Geometry: final body of the model. Coordinates: model frame, mm. A direction names the side the tool comes from. Give positions to 0.01 mm unless a question says otherwise; leave off trailing zeros. Loops run counter-clockwise (first coordinate to the right, second up) from the corner with the lowest first, then second, coordinate; pieces in that order, holes last. Notation, with made-up numbers: (-6, 65.25) -> (0, 65.25) arc R18 ccw to (0, 73.25) -> close; hole circle Ø5 at (6.5, 26.25). An arc over 180 degrees is marked (long way). Answer in a Markdown table with one row per item. Add a question column.
1) First-contact query: P1, Ø18, axis at x = -15.5, y = 5.5, coming from the +Z side; P2, Ø9.5, axis at y = -6, z = 10, coming from the +X side; P3, Ø2, axis at y = -13.5, z = 29, coming from the -X side; P4, Ø1.2, axis at x = -25.5, y = 16, coming from the +Z side. Flat tips, straight axial feed; report the tip coordinate or a pass-through.
2) Line query: line 1 (Y direction, x = 22, z = 10); line 2 (Z direction, x = 23, y = 6); line 3 (Z direction, x = 21.25, y = -6). Output: solid intervals per line, ascending. Write a range as from..to.
3) Section query B-B (x = 12.5). Return the cut outline in (y, z), plus the area to 3 significant figures.
4) Section query C-C (z = 10). Return the cut outline in (x, y), plus the area to 3 significant figures.
5) Section query A-A (y = 6). Give the number of separate pieces and of enclosed holes in the cut face, plus the area to 4 significant figures.
6) Draft query along Z for faces 1 (the cylindrical face through (23.49, -7.15, 22.88)), 2 (the flat face through (1.5, 0, 16)). Return one class per face: +Z half, -Z half, draft (parallel to the pull), parting line (faces both ways), or undercut.
7) Section query D-D (x = 18.5). Return the cut outline in (y, z), plus the area to 3 significant figures.
8) Access query for faces 3 (the flat face through (-11, -8, 16)), 4 (the flat face through (-27.5, 0, 16)), 5 (the flat face through (-3, -18, 16)), 6 (the cylindrical face through (21.49, 5.35, 24.93)). Directions: +Z, -Z, +X, -X, +Y, -Y. A direction counts if a zero-diameter tool reaches every point of the face in a straight line with its end or side. Return the directions, or none.
```python
from build123d import *

# Parameters (mm, degrees)
SKETCH005_W     = 64
SKETCH005_H     = 35.4
PAD_DEPTH       = 4
SKETCH_R        = 3
POCKET_DEPTH    = 2
SKETCH006_R     = 1.45
POCKET001_DEPTH = 5
SKETCH007_W     = 36
SKETCH007_H     = 3
PAD001_DEPTH    = 48
SKETCH008_R     = 1
SKETCH008_W     = 16
SKETCH008_H     = 24.5
POCKET002_DEPTH = 5


with BuildPart() as part:
    # Sketch005 → Pad (new body)
    with BuildSketch(Plane.YZ.offset(20.5)):
        with Locations((0, 17.7)):
            Rectangle(SKETCH005_W, SKETCH005_H)
    extrude(amount=PAD_DEPTH)

    # Sketch (on Face5 of Pad) → Pocket (cut)
    with BuildSketch(Plane(origin=(20.5, 0, 0), x_dir=(0, 1, 0), z_dir=(-1, 0, 0))):
        with Locations((6, -22)):
            Circle(SKETCH_R)
        with Locations((-6, -22)):
            Circle(SKETCH_R)
        with Locations((6, -10)):
            Circle(SKETCH_R)
        with Locations((-6, -10)):
            Circle(SKETCH_R)
    extrude(amount=-POCKET_DEPTH, mode=Mode.SUBTRACT)

    # Sketch006 (on Face4 of Pocket) → Pocket001 (cut)
    with BuildSketch(Plane(origin=(20.5, 0, 0), x_dir=(0, 1, 0), z_dir=(-1, 0, 0))):
        with Locations((6, -22)):
            Circle(SKETCH006_R)
        with Locations((-6, -22)):
            Circle(SKETCH006_R)
        with Locations((6, -10)):
            Circle(SKETCH006_R)
        with Locations((-6, -10)):
            Circle(SKETCH006_R)
    extrude(amount=-POCKET001_DEPTH, mode=Mode.SUBTRACT)

    # Sketch007 (on Face4 of Pocket001) → Pad001 (join)
    with BuildSketch(Plane(origin=(20.5, 0, 0), x_dir=(0, 1, 0), z_dir=(-1, 0, 0))):
        with Locations((0, -16)):
            Rectangle(SKETCH007_W, SKETCH007_H)
    extrude(amount=PAD001_DEPTH)

    # Sketch008 (on Face9 of Pad001) → Pocket002 (cut)
    with BuildSketch(Plane(origin=(20.5, 0, 14.5), x_dir=(0, 1, 0), z_dir=(0, 0, -1))):
        with Locations((16, -46)):
            Circle(SKETCH008_R)
        with Locations((-16, -46)):
            Circle(SKETCH008_R)
        with Locations((16, -2)):
            Circle(SKETCH008_R)
        with Locations((-16, -2)):
            Circle(SKETCH008_R)
        Polygon((12.65, -28), (10.15, -28), (10.15, -16), (-10.15, -16), (-10.15, -28), (-12.65, -28), (-12.65, -7), (-10.15, -7), (-10.15, -4), (10.15, -4), (10.15, -7), (12.65, -7), align=None)
        with Locations((0, -31.25)):
            Rectangle(SKETCH008_W, SKETCH008_H)
    extrude(amount=-POCKET002_DEPTH, mode=Mode.SUBTRACT)


solid = part.part
```
Evaluation:
| question | item | result |
|---|---|---|
| 1 | P1 | z = 17.5 |
| 1 | P2 | x = 24.5 |
| 1 | P3 | x = 20.5 |
| 1 | P4 | through |
| 2 | line 1 | -32..-9, -3..3, 9..32 |
| 2 | line 2 | 0..8.55, 11.45..20.55, 23.45..35.4 |
| 2 | line 3 | 0..7, 13..19, 25..35.4 |
| 3 | outline | (-18, 14.5) -> (-12.65, 14.5) -> (-12.65, 17.5) -> (-18, 17.5) -> close; (12.65, 14.5) -> (18, 14.5) -> (18, 17.5) -> (12.65, 17.5) -> close |
| 3 | area | 32.1 mm² |
| 4 | outline | (20.5, -32) -> (24.5, -32) -> (24.5, -7.45) -> (22.5, -7.45) -> (22.5, -9) -> (20.5, -9) -> close; (20.5, -3) -> (22.5, -3) -> (22.5, -4.55) -> (24.5, -4.55) -> (24.5, 4.55) -> (22.5, 4.55) -> (22.5, 3) -> (20.5, 3) -> close; (20.5, 9) -> (22.5, 9) -> (22.5, 7.45) -> (24.5, 7.45) -> (24.5, 32) -> (20.5, 32) -> close |
| 4 | area | 220 mm² |
| 5 | separate pieces | 5 |
| 5 | enclosed holes | 0 |
| 5 | area | 140.5 mm² |
| 6 | face 1 | undercut |
| 6 | face 2 | draft |
| 7 | outline | (-18, 14.5) -> (-17, 14.5) -> (-17, 17.5) -> (-18, 17.5) -> close; (-15, 14.5) -> (15, 14.5) -> (15, 17.5) -> (-15, 17.5) -> close; (17, 14.5) -> (18, 14.5) -> (18, 17.5) -> (17, 17.5) -> close |
| 7 | area | 96.0 mm² |
| 8 | face 3 | +Z, -Z |
| 8 | face 4 | +Z, -Z, -X, +Y, -Y |
| 8 | face 5 | +Z, -Z, -X, -Y |
| 8 | face 6 | -X |
